The listing builds one solid part. Answer for the finished solid, in the listing's coordinates (mm). Face numbers are marked on the shaded views. A direction names the side the tool comes from. Round coordinates to 2 decimals unless told otherwise and drop trailing zeros. Write each loop counter-clockwise with the first axis right and the second up, starting at its lowest first coordinate (ties: lowest second). Pieces come first, ordered by that corner, then holes. Notation, with made-up numbers: (29, 48.25) - (39, 48.25) arc R27 ccw to (39, 70.25) - close; hole circle Ø8 at (41, 78). An arc over 180 degrees is marked (long way). Return JSON: item names as keys, results as strings. Group by question number.
(1) Which of the six approach directions +Z, -Z, +X, -X, +Y, -Y give full straight-line access (tool end or side, diameter ignored) to the marked faces 1, 2 and 3?
(2) Section A-A, the plane z = -5 is taken. Write down the section's boundary in (x, y) (3 decimals), then the cut area to 3 significant figures.
(3) Section B-B, the plane y = 12 is taken. Write down the section's boundary in (x, z), then the cut area to 3 significant figures.
(4) Determine the mould class of the marked faces 4, 5 and 6 for opening direction Z: +Z half, -Z half, draft (parallel to the pull), parting line (faces both ways), or undercut.
(5) Section C-C, the plane z = -2.25 is taken. Write down the section's boundary in (x, y) (3 decimals).
(6) Find the intervals of material crossed by line 1 along Y through (x, z) = (3.1, -5); line 2 along Y through (x, z) = (1.9, -6); line 3 along Y through (x, z) = (2.85, -2.5), in increasing order. Write a range as [from, to].
(7) Section D-D, the plane x = 4.2 is taken. Write down the section's boundary in (y, z).
(8) Each of these flat-tipped pins is pushed along its axis until it touches: pin 1 (0.8 mm diameter, centred on y = -2.5, z = -5, fed in from -X) (3 decimals); pin 2 (0.5 mm diameter, centred on x = 2.5, y = -1.5, fed in from -Z); pin 3 (3 mm diameter, centred on y = 9.5, z = -5, fed in from -X); pin 4 (1 mm diameter, centred on y = -1.5, z = -2, fed in from +X) (3 decimals). Where does it stop, or does it pass through?
```python
from build123d import *

# Parameters (mm, degrees)
SKETCH_1_W          = 4.5
SKETCH_1_H          = 10
EXTRUDE_1_DEPTH     = 9
SKETCH_2_W          = 2.25
SKETCH_2_H          = 10
EXTRUDE_2_DEPTH     = 6
SKETCH_3_R          = 1.6
CUT_EXTRUDE_1_DEPTH = 19.167622299
SKETCH_4_W          = 0.65
SKETCH_4_H          = 1.3
SKETCH_4_H_2        = 1.5
EXTRUDE_3_DEPTH     = 4


with BuildPart() as part:
    # Эскиз1 → Бобышка-Вытянуть1 (new body)
    with BuildSketch(Plane(origin=(0, 0, 0), x_dir=(1, 0, 0), z_dir=(0, 1, 0))):
        with Locations((2.25, 5)):
            Rectangle(SKETCH_1_W, SKETCH_1_H)
    extrude(amount=EXTRUDE_1_DEPTH)

    # Эскиз2 → Бобышка-Вытянуть2 (add)
    with BuildSketch(Plane(origin=(0, 9, 0), x_dir=(1, 0, 0), z_dir=(0, 1, 0))):
        with Locations((3.375, 5)):
            Rectangle(SKETCH_2_W, SKETCH_2_H)
    extrude(amount=EXTRUDE_2_DEPTH)

    # Эскиз3 → Вырез-Вытянуть1 (cut, through all)
    with BuildSketch(Plane.ZY.offset(-2.25)):
        with Locations((-5, 12)):
            Circle(SKETCH_3_R)
    extrude(amount=-CUT_EXTRUDE_1_DEPTH, mode=Mode.SUBTRACT)

    # Эскиз4 → Бобышка-Вытянуть3 (add)
    with BuildSketch(Plane.XZ):
        with Locations((2.25, -1.81)):
            Rectangle(SKETCH_4_W, SKETCH_4_H)
        with Locations((2.25, -5)):
            Rectangle(SKETCH_4_W, SKETCH_4_H_2)
        with Locations((2.25, -8.19)):
            Rectangle(SKETCH_4_W, SKETCH_4_H)
    extrude(amount=EXTRUDE_3_DEPTH)


solid = part.part
```
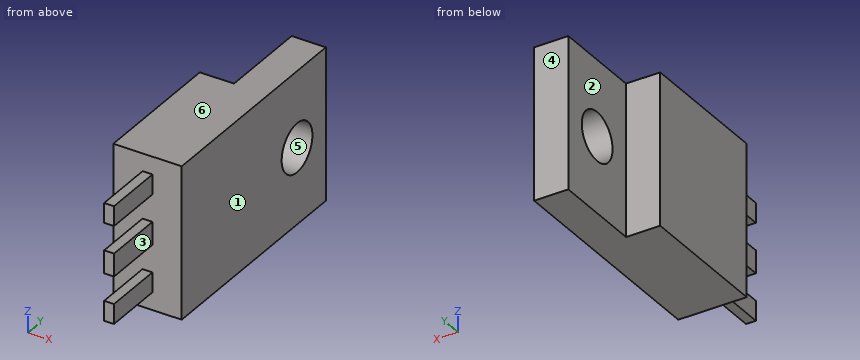
Working result:
{
 "1": {"face 1": "+Z, -Z, +X, +Y, -Y", "face 2": "+Z, -Z, -X, +Y", "face 3": "+Z, -Z, +X, -Y"},
 "2": {"outline": "(0, 0) - (1.925, 0) - (1.925, -4) - (2.575, -4) - (2.575, 0) - (4.5, 0) - (4.5, 10.4) - (2.25, 10.4) - (2.25, 9) - (0, 9) - close; (2.25, 13.6) - (4.5, 13.6) - (4.5, 15) - (2.25, 15) - close", "area": "49.4 mm^2"},
 "3": {"outline": "(2.25, -10) - (4.5, -10) - (4.5, -6.6) - (2.25, -6.6) - close; (2.25, -3.4) - (4.5, -3.4) - (4.5, 0) - (2.25, 0) - close", "area": "15.3 mm^2"},
 "4": {"face 4": "draft", "face 5": "undercut", "face 6": "+Z half"},
 "5": {"outline": "(0, 0) - (1.925, 0) - (1.925, -4) - (2.575, -4) - (2.575, 0) - (4.5, 0) - (4.5, 15) - (2.25, 15) - (2.25, 9) - (0, 9) - close"},
 "6": {"line 1": "y = [0, 10.4], [13.6, 15]", "line 2": "y = [0, 9]", "line 3": "y = [0, 15]"},
 "7": {"outline": "(0, -10) - (15, -10) - (15, 0) - (0, 0) - close; hole circle Ø3.2 at (12, -5)"},
 "8": {"pin 1": "stops at x = 1.925", "pin 2": "stops at z = -8.84", "pin 3": "stops at x = 0", "pin 4": "stops at x = 2.575"}
}
